The model under review builds one solid part; all positions refer to its coordinate system, in mm. A direction names the side the tool comes from. Round coordinates to 2 decimals unless told otherwise and drop trailing zeros. Write each loop counter-clockwise with the first axis right and the second up, starting at its lowest first coordinate (ties: lowest second). Pieces come first, ordered by that corner, then holes. Notation, with made-up numbers: (-17.75, -35) - (-8.75, -35) arc R18 cw to (-8.75, -26) - close; hole circle Ø11 at (-33.5, -17.75). An arc over 180 degrees is marked (long way). Use one line per item in the form item = value.
from build123d import *

# Parameters (mm, degrees)
F0_R     = 14.3239448783
F0_R_2   = 2.5
F2_DEPTH = 3
F3_DEPTH = 3
F4_COUNT = 30
F4_ANGLE = 348


with BuildPart() as f2:
    # F0 (on Top) → F2 (new body)
    with BuildSketch(Plane.XY):
        Circle(F0_R)
        Circle(F0_R_2, mode=Mode.SUBTRACT)
    extrude(amount=F2_DEPTH)

    # F1 (on face) → F3 (join)
    with BuildSketch(Plane.XY):
        with BuildLine():
            ThreePointArc((-1, 14.2889956566), (0, 14.3239448783), (1, 14.2889956566))
            Line((1, 14.2889956566), (0.5, 15.7889956566))
            Line((0.5, 15.7889956566), (-0.5, 15.7889956566))
            Line((-0.5, 15.7889956566), (-1, 14.2889956566))
        make_face()
    extrude(amount=F3_DEPTH)

    # F4: F2 ×30 about axis
    f4_axis = Axis((0, 0, 0), (0, 0, -1))


with BuildPart() as f2_1:
    add(f2.part)
    for i in range(1, F4_COUNT):
        add(f2.part.rotate(f4_axis, i * F4_ANGLE / (F4_COUNT - 1)))


solid = f2_1.part
(1) Machinability: for faces 1 (the flat face through (-8.22, 12.6, 1.48)), 2 (the flat face through (-5.44, -14.05, 1.48)), 3 (the cylindrical face through (-14.01, 2.98, 1.48)), 4 (the flat face through (-6.8, -13.4, 1.5)), 5 (the flat face through (14.889, 2.316, 1.479)), which of the approach directions +Z, -Z, +X, -X, +Y, -Y give a long, thin tool a straight path to every point of the face, cutting with its end or side? Answer none if there is none.
Geometry results:
face_1 = +Z, -Z, +Y
face_2 = +Z, -Z, -Y
face_3 = +Z, -Z, -X
face_4 = +Z, -Z
face_5 = +Z, -Z, +X
(2) Add section A-A on x = 0. Write out the cut boundary in (y, z), then the cut area to 3 significant figures.
Geometry results:
outline = (-15.79, 0) - (-2.5, 0) - (-2.5, 3) - (-15.79, 3) - close; (2.5, 0) - (15.79, 0) - (15.79, 3) - (2.5, 3) - close
area = 79.7 mm2
(3) Add section B-B on y = 0. Write out the cut boundary in (x, z), then the cut area to 3 significant figures.
Geometry results:
outline = (-14.32, 0) - (-2.5, 0) - (-2.5, 3) - (-14.32, 3) - close; (2.5, 0) - (14.32, 0) - (14.32, 3) - (2.5, 3) - close
area = 70.9 mm2
(4) Insertion check: P1, Ø1, axis at y = -5.5, z = 2, coming from the -X side. The pin has a flat end and moves straight along its axis. Give the tip position at first contact, or say it passes through.
Geometry results:
P1 = -14.98
(5) Add section C-C on y = -7. Write out the cut boundary in (x, z), then the cut area to 3 significant figures.
Geometry results:
outline = (-13.51, 0) - (13.51, 0) - (13.51, 3) - (-13.51, 3) - close
area = 81.1 mm2
(6) To check wall thickness, follow L1, parallel to X at y = 0, z = 1.8; L2, parallel to Y at x = 0, z = 1.9; L3, parallel to Y at x = -12, z = 2.75. State the ranges of each line that lie inside material, in increasing order.
Geometry results:
L1 = -14.32 to -2.5, 2.5 to 14.32
L2 = -15.79 to -2.5, 2.5 to 15.79
L3 = -10.27 to -10.07, -8.04 to 8.04, 10.07 to 10.27
(7) The part is to be moulded in two halves that separate along Y. For faces 6 (the cylindrical face through (14.324, -0.007, 1.479)), 7 (the flat face through (5.424, -14.036, 1.479)), 8 (the flat face through (0, 15.789, 1)), say which applies: +Y half, -Y half, draft (parallel to the pull), parting line (faces both ways), or undercut.
Geometry results:
face_6 = undercut
face_7 = -Y half
face_8 = +Y half
